```python
from build123d import *

# Parameters (mm, degrees)
F1_DEPTH      = 20
F2_R          = 6
F3_DEPTH      = 40
F3_DEPTH_BACK = 40
F4_R          = 12
F5_DEPTH      = 20
F7_R          = 2.5
F8_DEPTH      = 25
F9_T1_DEPTH   = 20


# Not quite as in the source:
# - a fillet or chamfer that OpenCascade refuses, or shapes differently, is made with other operations: its cross-section is extruded or revolved along the edge and cut away or added
# - a feature names something its author has since deleted; it is built from what else it names


with BuildPart() as f1:
    # F0 (on Front) → F1 (new body)
    with BuildSketch(Plane.XZ):
        with BuildLine():
            ThreePointArc((-12, 33.941125497), (-29.3938769134, 20.7846096908), (-36, 0))
            Line((-36, 0), (-30, 0))
            Line((-30, 0), (-24, 0))
            ThreePointArc((-24, 0), (0, 24), (24, 0))
            Line((24, 0), (30, 0))
            Line((30, 0), (36, 0))
            ThreePointArc((36, 0), (29.3938769134, 20.7846096908), (12, 33.941125497))
            Line((12, 33.941125497), (12, 43.941125497))
            Line((12, 43.941125497), (-12, 43.941125497))
            Line((-12, 43.941125497), (-12, 33.941125497))
        make_face()
        Polygon((-30, 0), (-36, 0), (-40, 0), (-40, -28.374), (-40, -36), (-24, -36), (-24, -33.2482792437), (-30, -28.374), align=None)
        Polygon((36, 0), (30, 0), (30, -28.374), (24, -33.2482792437), (24, -36), (40, -36), (40, -28.374), (40, 0), align=None)
    extrude(amount=F1_DEPTH)

    # F2 (on face) → F3 (join, two sides)
    with BuildSketch(Plane.XY.offset(43.941125497)) as f3_sk:
        with Locations((0, -10)):
            Circle(F2_R)
    extrude(amount=F3_DEPTH)
    extrude(f3_sk.sketch, amount=-F3_DEPTH_BACK)

    # F4 (on face) → F5 (join)
    with BuildSketch(Plane.XY.offset(83.941125497)):
        with Locations((0, -10)):
            Circle(F4_R)
    extrude(amount=F5_DEPTH)

    # F7 (on offset) → F8 (cut)
    with BuildSketch(Plane.YZ.offset(12)):
        with Locations((-10.1158004254, 93.941125497)):
            Circle(F7_R)
    extrude(amount=-F8_DEPTH, mode=Mode.SUBTRACT)

    # F9: fillet of radius 4 on 4 edges, made by hand

    # F9_s2 → F9_t1 (join)
    with BuildSketch(Plane.XZ):
        with BuildLine():
            add(Edge.make_bspline(
                [(35.8195477358, 3.6), (36.1813613493, 0), (39.7994974843, 0)],
                knots=[0, 0, 0, 1, 1, 1], degree=2, weights=[1, 1, 1]))
            Line((39.7994974843, 0), (36, 0))
            ThreePointArc((36, 0), (35.954858632, 1.8022599022), (35.8195477358, 3.6))
        make_face()
        with BuildLine():
            add(Edge.make_bspline(
                [(-35.8195477358, 3.6), (-36.1813613493, 0), (-39.7994974843, 0)],
                knots=[0, 0, 0, 1, 1, 1], degree=2, weights=[1, 1, 1]))
            Line((-39.7994974843, 0), (-36, 0))
            ThreePointArc((-36, 0), (-35.954858632, 1.8022599022), (-35.8195477358, 3.6))
        make_face()
        with BuildLine():
            add(Edge.make_bspline(
                [(-12, 36.6606055596), (-12, 34.0419908768), (-14.4, 32.9945450037)],
                knots=[0, 0, 0, 1, 1, 1], degree=2, weights=[1, 1, 1]))
            ThreePointArc((-14.4, 32.9945450037), (-13.2084822617, 33.4893415334), (-12, 33.941125497))
            Line((-12, 33.941125497), (-12, 36.6606055596))
        make_face()
        with BuildLine():
            add(Edge.make_bspline(
                [(12, 36.6606055596), (12, 34.0419908768), (14.4, 32.9945450037)],
                knots=[0, 0, 0, 1, 1, 1], degree=2, weights=[1, 1, 1]))
            ThreePointArc((14.4, 32.9945450037), (13.2084822617, 33.4893415334), (12, 33.941125497))
            Line((12, 33.941125497), (12, 36.6606055596))
        make_face()
    extrude(amount=F9_T1_DEPTH)


solid = f1.part
```
Could you check a few things on this model? Use its own coordinates, in mm. A direction names the side the tool comes from. Give positions to 0.01 mm unless a question says otherwise; leave off trailing zeros. Loops run counter-clockwise (first coordinate to the right, second up) from the corner with the lowest first, then second, coordinate; pieces in that order, holes last. Notation, with made-up numbers: (-2.5, 87) -> (5.5, 87) arc R27 cw to (5.5, 120) -> close; hole circle Ø6 at (-19, 33). An arc over 180 degrees is marked (long way). Put each result on its own line as item: value.
(1) Imagine slicing it at D-D on x = 0. Write out the boundary of the cut face in (y, z).
Computed:
outline: (-22, 83.94) -> (-16, 83.94) -> (-16, 43.94) -> (-20, 43.94) -> (-20, 24) -> (-16, 24) -> (-16, 3.94) -> (-4, 3.94) -> (-4, 24) -> (0, 24) -> (0, 43.94) -> (-4, 43.94) -> (-4, 83.94) -> (2, 83.94) -> (2, 103.94) -> (-22, 103.94) -> close; hole circle Ø5 at (-10.12, 93.94)
(2) Thinking about a two-plate mould opening in Z: for faces 1 (the face through (0, -10, 3.941)), 2 (the face through (0, -10, 103.941)), 3 (the face through (30, -10, -14)), 4 (the face through (2, -4, 83.941)), which applies, pulls with the +Z half, pulls with the -Z half, needs draft (parallel to the pull), parting line crosses it, or undercut?
Computed:
face 1: pulls with the -Z half
face 2: pulls with the +Z half
face 3: undercut
face 4: undercut
(3) For faces 5 (the face through (27.04, -9.86, -30.78)), 6 (the face through (0, -3, 43.941)), 7 (the face through (-24, -10, -35)), which set-ups out of +Z, -Z, +X, -X, +Y, -Y let a thin tool reach every point of the face, with its end or its side?
Computed:
face 5: +Y, -Y
face 6: none
face 7: -Z, +Y, -Y
(4) Imagine slicing it at B-B on x = 27. Write out the boundary of the cut face in (y, z), plus the area to 3 significant figures.
Computed:
outline: (-20, -36) -> (0, -36) -> (0, -30.81) -> (-20, -30.81) -> close; (-20, 0) -> (0, 0) -> (0, 23.81) -> (-20, 23.81) -> close
area: 580 mm^2
(5) I'm going to push flat-ended pins straight in: pin 1 Ø3 at (x, y) = (6.5, -18.5) entering from -Z; pin 2 Ø9.5 at (x, y) = (2.5, -8) entering from -Z; pin 3 Ø8 at (y, z) = (-9.5, 39.5) entering from -X. Where does each tip first touch, or does it pass through?
Computed:
pin 1: z = 22.63
pin 2: z = 3.94
pin 3: x = -12.14
(6) Please list where these lines run through material, in increasing order: probe 1 along Y at (x, z) = (-35.5, -3); probe 2 along X at (y, z) = (-16.5, -27.5); probe 3 along Z at (x, y) = (5.5, -3.5). Write a range as [from, to].
Computed:
probe 1: [-20, 0]
probe 2: [-40, -30], [30, 40]
probe 3: [23.36, 43.94], [83.94, 103.94]
(7) Imagine slicing it at C-C on z = 8.5. Write out the boundary of the cut face in (x, y).
Computed:
outline: (-34.98, -20) -> (-22.44, -20) -> (-22.44, 0) -> (-34.98, 0) -> close; circle Ø12 at (0, -10); (22.44, -20) -> (34.98, -20) -> (34.98, 0) -> (22.44, 0) -> close
(8) Imagine slicing it at A-A on z = -11.5. Write out the boundary of the cut face in (x, y), plus the area to 3 significant figures.
Computed:
outline: (-40, -20) -> (-30, -20) -> (-30, 0) -> (-40, 0) -> close; (30, -20) -> (40, -20) -> (40, 0) -> (30, 0) -> close
area: 400 mm^2
